Read the model definition and answer for the solid it produces. Units are mm, in the model's axes. A direction names the side the tool comes from. Coordinates: 2 decimals unless noted, no trailing zeros. Loops run counter-clockwise (first coordinate to the right, second up) from the corner with the lowest first, then second, coordinate; pieces in that order, holes last. Notation, with made-up numbers: (13.25, 83) -> (45.25, 83) arc R11 cw to (45.25, 95) -> close; hole circle Ø1 at (75, -22). An arc over 180 degrees is marked (long way). Answer in a Markdown table with one row per item.
```python
from build123d import *

# Parameters (mm, degrees)
SKETCH1_W                           = 10
SKETCH1_H                           = 5
SKETCH1_W_2                         = 5
SKETCH1_H_2                         = 40
BOSS_EXTRUDE1_DEPTH                 = 20
SKETCH3_W                           = 15
SKETCH3_H                           = 5
BOSS_EXTRUDE2_DEPTH                 = 20.3
CHAMFER2_SIZE                       = 7.5
SKETCH4_W                           = 5
SKETCH4_H                           = 15
BOSS_EXTRUDE3_DEPTH                 = 15
FILLET1_R                           = 7.5
F_5_5_5_5_DIAMETER_HOLE1_AT_2_COUNT = 2
F_5_5_5_5_DIAMETER_HOLE1_AT_2_PITCH = 12.5
FILLET2_R                           = 2


with BuildPart() as part:
    # Sketch1 → Boss-Extrude1 (new body)
    with BuildSketch(Plane(origin=(0, 0, 0), x_dir=(0, 0, -1), z_dir=(1, 0, 0))):
        with Locations((-5, 17.5)):
            Rectangle(SKETCH1_W, SKETCH1_H)
        with Locations((2.5, 0)):
            Rectangle(SKETCH1_W_2, SKETCH1_H_2)
    extrude(amount=BOSS_EXTRUDE1_DEPTH)

    # Sketch3 → Boss-Extrude2 (add)
    with BuildSketch(Plane(origin=(0, 0, 0), x_dir=(0, 0, -1), z_dir=(1, 0, 0))):
        with Locations((-2.5, 17.5)):
            Rectangle(SKETCH3_W, SKETCH3_H)
    extrude(amount=-BOSS_EXTRUDE2_DEPTH)

    # Chamfer2
    chamfer2_edges = [part.edges().sort_by_distance(p)[0] for p in [
        (10, 15, 0),
    ]]
    chamfer(chamfer2_edges, length=CHAMFER2_SIZE)

    # Sketch4 → Boss-Extrude3 (add)
    with BuildSketch(Plane(origin=(0, 20, 0), x_dir=(1, 0, 0), z_dir=(0, 1, 0))):
        with Locations((-17.8, -2.5)):
            Rectangle(SKETCH4_W, SKETCH4_H)
        with Locations((2.5, -2.5)):
            Rectangle(SKETCH4_W, SKETCH4_H)
    extrude(amount=BOSS_EXTRUDE3_DEPTH)

    # Fillet1
    # the kernel refuses this fillet: 7.5 mm, written as the material it adds along each edge
    with BuildSketch(Plane(origin=(0, 15, 7.5), x_dir=(0, -0.7071067811865472, -0.7071067811865479), z_dir=(1, 0, 0))) as fillet1_piece_1:
        with BuildLine():
            CenterArc((3.068709481, -7.5), FILLET1_R, 90, 40.155443777)
            Line((-1.767766953, -1.767766953), (0, 0))
            Line((0, 0), (3.068709481, 0))
        make_face()
    extrude(amount=20)
    with BuildSketch(Plane(origin=(0, 15, -5), x_dir=(0, -1, 0), z_dir=(0, 0, 1))) as fillet1_piece_2_section:
        with BuildLine():
            CenterArc((FILLET1_R, -FILLET1_R), FILLET1_R, 90, 90)
            Line((0, -FILLET1_R), (0, 0))
            Line((0, 0), (FILLET1_R, 0))
        make_face()
    fillet1_piece_2 = extrude(amount=31.25, mode=Mode.PRIVATE)
    fillet1_piece_2 = split(fillet1_piece_2, bisect_by=Plane(origin=(0, 8.75, 1.25), z_dir=(0, 0.7071067811865477, -0.7071067811865474)), keep=Keep.TOP, mode=Mode.PRIVATE)
    add(fillet1_piece_2)
    with BuildSketch(Plane(origin=(0, 15, -5), x_dir=(0, -1, 0), z_dir=(0, 0, 1))) as fillet1_piece_3a_section:
        with BuildLine():
            CenterArc((FILLET1_R, -FILLET1_R), FILLET1_R, 90, 90)
            Line((0, -FILLET1_R), (0, 0))
            Line((0, 0), (FILLET1_R, 0))
        make_face()
    fillet1_piece_3a = extrude(amount=31.25, mode=Mode.PRIVATE)
    fillet1_piece_3a = split(fillet1_piece_3a, bisect_by=Plane(origin=(0, 15, 10), z_dir=(0, 0, -1)), keep=Keep.TOP, mode=Mode.PRIVATE)
    fillet1_piece_3a = split(fillet1_piece_3a, bisect_by=Plane(origin=(0, 8.75, 1.25), z_dir=(0, -0.7071067811865477, 0.7071067811865474)), keep=Keep.TOP, mode=Mode.PRIVATE)
    with BuildSketch(Plane(origin=(-7.671773702, 15, 7.5), x_dir=(0, -0.7071067811865472, -0.7071067811865479), z_dir=(1, 0, 0))) as fillet1_piece_3b_section:
        with BuildLine():
            CenterArc((3.068709481, -7.5), FILLET1_R, 90, 40.155443777)
            Line((-1.767766953, -1.767766953), (0, 0))
            Line((0, 0), (3.068709481, 0))
        make_face()
    fillet1_piece_3b = extrude(amount=27.671773702, mode=Mode.PRIVATE)
    fillet1_piece_3b = split(fillet1_piece_3b, bisect_by=Plane(origin=(0, 15, 7.5), z_dir=(-1, 0, 0)), keep=Keep.TOP, mode=Mode.PRIVATE)
    fillet1_piece_3 = fillet1_piece_3a & fillet1_piece_3b
    add(fillet1_piece_3)

    # Sketch9 → Ø5.5 (5.5) Diameter Hole1 (revolve, cut)
    with BuildSketch(Plane(origin=(10, 0, 0), x_dir=(0, -1, 0), z_dir=(1, 0, 0))):
        Polygon((0, 0), (0, 5), (2.75, 5), (2.75, 0.301776695), (2.875, 0), align=None)
    f_5_5_5_5_diameter_hole1 = revolve(axis=Axis((10, 0, 6.35), (0, 0, -1)), mode=Mode.SUBTRACT)

    # Ø5.5 (5.5) Diameter Hole1 at 2: Ø5.5 (5.5) Diameter Hole1 ×2
    with Locations(*[(0, -i * F_5_5_5_5_DIAMETER_HOLE1_AT_2_PITCH, 0) for i in range(1, F_5_5_5_5_DIAMETER_HOLE1_AT_2_COUNT)]):
        add(f_5_5_5_5_diameter_hole1, mode=Mode.SUBTRACT)

    # Sketch12 → Ø4.0 (4) Diameter Hole1 (revolve, cut)
    with BuildSketch(Plane(origin=(-20.3, 27.5, 2.5), x_dir=(0, 0, 1), z_dir=(0, 1, 0))):
        Polygon((0, 0), (0, 5), (2, 5), (2, 0.301776695), (2.125, 0), align=None)
    f_4_0_4_diameter_hole1 = revolve(axis=Axis((-26.65, 27.5, 2.5), (1, 0, 0)), mode=Mode.SUBTRACT)

    # Mirror1: Ø4.0 (4) Diameter Hole1 across plane
    add(f_4_0_4_diameter_hole1.mirror(Plane(origin=(-7.65, 0, 0), x_dir=(0, 0, 1), z_dir=(1, 0, 0))), mode=Mode.SUBTRACT)

    # Fillet2
    fillet2_edges = [part.edges().sort_by_distance(p)[0] for p in [
        (20, -20, -2.5),
        (-20.3, 15, 2.5),
        (20, 20, 2.5),
        (-17.8, 35, -5),
        (-17.8, 35, 10),
        (5, 20, 2.5),
        (2.5, 35, 10),
        (2.5, 35, -5),
        (0, -20, -2.5),
    ]]
    fillet(fillet2_edges, radius=FILLET2_R)


solid = part.part
```
1. A cutting plane is placed at B-B on x = 10. Give the vertices of the cut face in (y, z) (3 decimals), and give its area (3 significant figures).
A:
| item | result |
|---|---|
| outline | (-20, -5) -> (-15.25, -5) -> (-15.25, -0.302) -> (-15.375, 0) -> (-20, 0) -> close; (-9.75, -5) -> (-2.75, -5) -> (-2.75, -0.302) -> (-2.875, 0) -> (-9.625, 0) -> (-9.75, -0.302) -> close; (2.75, -5) -> (20, -5) -> (20, 10) -> (15, 10) arc R7.5 cw to (12.83, 5.33) -> (7.5, 0) -> (2.875, 0) -> (2.75, -0.302) -> close |
| area | 224 mm2 |
2. Find the intervals of material crossed by probe 1 along Y at (x, z) = (10, -3.2); probe 2 along Y at (x, z) = (1.6, 2.5); probe 3 along Z at (x, y) = (-16.9, 27.5), in increasing order.
A:
| item | result |
|---|---|
| probe 1 | y = -20 to -15.25, -9.75 to -2.75, 2.75 to 20 |
| probe 2 | y = 10 to 25.5, 29.5 to 35 |
| probe 3 | z = -5 to 0.5, 4.5 to 10 |
3. A cutting plane is placed at A-A on y = 24. Give the vertices of the cut face in (x, z).
A:
| item | result |
|---|---|
| outline | (-20.3, -5) -> (-15.3, -5) -> (-15.3, 10) -> (-20.3, 10) -> close; (0, -5) -> (5, -5) -> (5, 10) -> (0, 10) -> close |
4. A tool of negligible diameter and unlimited length cuts with its end or side. For faces 1 (the flat face through (-8, 20, 3)), 2 (the flat face through (13, 20, 3)), 3 (the flat face through (0, 18, 10)), from which of +Z, -Z, +X, -X, +Y, -Y can it reach the whole face along a straight path? Write none if from no direction.
A:
| item | result |
|---|---|
| face 1 | +Z, -Z, +Y |
| face 2 | +Z, -Z, +X, +Y |
| face 3 | +Z, +X, -X, +Y, -Y |
5. The mould has two halves that part along Y. Classify faces 4 (the flat face through (10, -6, 0)), 5 (the cylindrical face through (-3.131, 13.596, 0.728)), 6 (the cylindrical face through (-17.682, 29.452, 2.066)), 7 (the cylindrical face through (11.05, -15.04, -2.62)): pulls with the +Y half, pulls with the -Y half, needs draft (parallel to the pull), parting line crosses it, or undercut.
A:
| item | result |
|---|---|
| face 4 | needs draft |
| face 5 | pulls with the -Y half |
| face 6 | undercut |
| face 7 | undercut |
6. A cutting plane is placed at C-C on z = 2.5. Give the vertices of the cut face in (x, y) (3 decimals).
A:
| item | result |
|---|---|
| outline | (-20.3, 17) arc R2 ccw to (-18.3, 15) -> (-7.5, 15) arc R7.5 cw to (-0.429, 10) -> (20, 10) -> (20, 18) arc R2 ccw to (18, 20) -> (7, 20) arc R2 cw to (5, 22) -> (5, 25.375) -> (4.698, 25.5) -> (0, 25.5) -> (0, 20) -> (-15.3, 20) -> (-15.3, 25.5) -> (-19.998, 25.5) -> (-20.3, 25.375) -> close; (-20.3, 29.625) -> (-19.998, 29.5) -> (-15.3, 29.5) -> (-15.3, 35) -> (-20.3, 35) -> close; (0, 29.5) -> (4.698, 29.5) -> (5, 29.625) -> (5, 35) -> (0, 35) -> close |
7. Given pin 1 Ø2 at (x, z) = (7.5, 3) entering from -Y; pin 2 Ø8 at (x, z) = (-12.5, 2) entering from +Y; pin 3 Ø6.5 at (x, y) = (10, 0) entering from +Z; pin 4 Ø1.5 at (x, z) = (7.5, 2) entering from -Y, each flat-ended and moving along its own axis, determine where each tip first touches the part or whether it passes through.
A:
| item | result |
|---|---|
| pin 1 | stops at y = 9.5 |
| pin 2 | stops at y = 35 |
| pin 3 | stops at z = 0 |
| pin 4 | stops at y = 8.75 |
8. A cutting plane is placed at D-D on y = 0. Give the vertices of the cut face in (x, z) (3 decimals).
A:
| item | result |
|---|---|
| outline | (0, -5) -> (7.25, -5) -> (7.25, -0.302) -> (7.125, 0) -> (0, 0) -> close; (12.75, -5) -> (20, -5) -> (20, 0) -> (12.875, 0) -> (12.75, -0.302) -> close |
